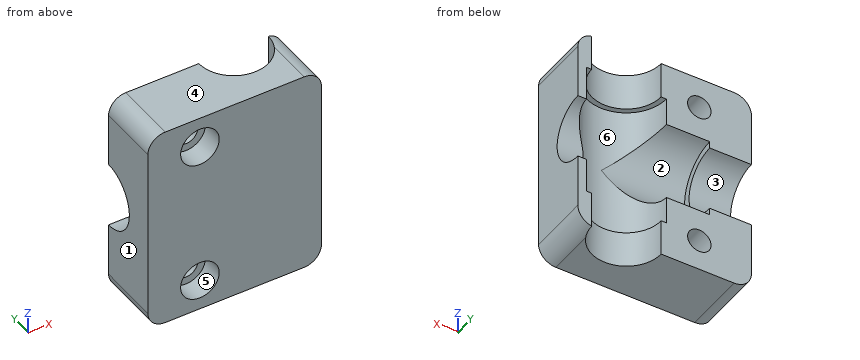
Autodesk Inventor part; units mm, degrees
ref_plane "Work Plane2" through (11, 18, -30) normal (1, 0, 0) x (0, 1, 0)
ref_plane "XZ Plane" through (0, 0, 0) normal (0, 1, 0) x (-1, 0, 0)
ref_plane "XY Plane" through (0, 0, 0) normal (0, 0, 1) x (1, 0, 0)
sketch "Sketch1" plane through (0, 0, 0) normal (0, 1, 0) x (-1, 0, 0)
  line L0 (-25, 30) -> (25, 30)
  line L1 (25, 30) -> (25, -30)
  line L2 (25, -30) -> (-25, -30)
  line L3 (-25, -30) -> (-25, 30)
  line L4 (-25, 30) -> (25, -30) construction
  line L5 (25, 30) -> (-25, -30) construction
  point P0 (0, 0)
  dimension "d0" = 50
  dimension "d1" = 60
extrude "Extrusion1" add sketch "Sketch1" along normal blind 18
sketch "Sketch2" plane through (25, 0, 30) normal (1, 0, 0) x (0, 0, -1)
  line L0 (60, 18) -> (0, 18)
  circle A0 centre (30, 18) radius 9.5
  point P0 (30, 0)
  point P1 (20.5, 18)
  point P2 (39.5, 18)
  dimension "d4" = 19
extrude "Extrusion2" cut sketch "Sketch2" against normal through all contours A0 L0 picked at (28.8771, 15.0391)
sketch "Sketch3" plane through (25, 0, -30) normal (0, 0, -1) x (-1, 0, 0)
  line L0 (0, 18) -> (50, 18)
  circle A0 centre (14, 18) radius 10
  point P0 (25, 0)
  point P1 (24, 18)
  point P2 (4, 18)
  dimension "d7" = 20
  dimension "d8" = 14
extrude "Extrusion3" cut sketch "Sketch3" against normal through all contours L0 A0 picked at (12.1065, 15.2567)
sketch "Sketch4" plane through (0, 0, 0) normal (0, 0, 1) x (1, 0, 0)
  arc A0 (1, 18) -> (21, 18) centre (11, 18) ccw
  circle A1 centre (11, 18) radius 11.5
  point P0 (0, 0)
  dimension "d11" = 23
extrude "Extrusion4" cut sketch "Sketch4" along normal mid plane 39
ref_plane "Work Plane2" through (11, 18, -30) normal (1, 0, 0) x (0, 1, 0)
sketch "Sketch5" plane through (11, 18, -30) normal (1, 0, 0) x (0, 1, 0)
  arc A0 (0, 39.5) -> (0, 20.5) centre (0, 30) ccw
  circle A1 centre (0, 30) radius 11.5
  point P0 (-18, 30)
  dimension "d14" = 23
extrude "Extrusion5" cut sketch "Sketch5" against normal blind 24
sketch "Sketch7" plane through (0, 0, 0) normal (0, -1, 0) x (1, 0, 0)
  line L0 (25, -30) -> (-25, -30)
  line L1 (-25, 30) -> (25, 30)
  line L2 (-25, -30) -> (-25, 30)
  point P0 (0, 0)
  point P1 (-10, -21)
  point P2 (-10, 21)
  dimension "d28" = 9
  dimension "d29" = 9
  dimension "d30" = 15
hole "Hole2" at (-10, 0, -21) at (-10, 0, 21) direction (0, 1, 0) diameter 6.756 end through all counterbore diameter 11.113 counterbore depth 6.35
fillet "Fillet1" radius 5 4 edges at (-25, 9, -30) (-25, 9, 30) (25, 9, 30) (25, 9, -30)
properties part number "Valve Block Bottom"
Source: CAD feature listing. Evaluate the final solid. Frame: model axes, mm. Face numbers are marked on the shaded views. A direction names the side the tool comes from. Give positions to 0.01 mm unless a question says otherwise; leave off trailing zeros. Order: outer loops, then holes, each group sorted by start corner. A loop starts at its lowest first (then second) coordinate and runs counter-clockwise, first axis right, second up.
(1) Section query D-D (y = 11.5). State how many separate pieces and enclosed holes the cut face has, plus the area to 3 significant figures.
(2) Material intervals for line 1 along Z through (x, y) = (-10, 3.5); line 2 along X through (y, z) = (4.5, -21); line 3 along Z through (x, y) = (-10, 9.75), sorted ascending.
(3) Pull-direction query (X, two-part tool) for the marked faces 1, 2 and 3; classes: +X half, -X half, draft (parallel to the pull), parting line (faces both ways), or undercut.
(4) Access query for the marked faces 4, 5 and 6. Directions: +Z, -Z, +X, -X, +Y, -Y. A direction counts if a zero-diameter tool reaches every point of the face in a straight line with its end or side. Return the directions, or none.
(5) Section query B-B (y = 2.5). Return the cut outline in (x, z).
(6) Section query A-A (z = -21). Return the cut outline in (x, y).
(7) Section query C-C (x = -10). Return the cut outline in (y, z), plus the area to 3 significant figures.
(8) Contact query for flat-ended pins moving along their axis: P1, Ø9, axis at y = 11.5, z = -5, coming from the +X side; P2, Ø9, axis at x = -10, z = 21, coming from the -Y side; P3, Ø1, axis at x = -12, z = -6.5, coming from the +Y side. Output: stop coordinate, or through.
Outcome:
1. separate pieces: 4
1. enclosed holes: 2
1. area: 1,340 mm2
2. line 1: z = -30 to -26.56, -15.44 to 15.44, 26.56 to 30
2. line 2: x = -25 to -15.56, -4.44 to 25
2. line 3: z = -30 to -24.38, -17.62 to -8.01, 8.01 to 17.62, 24.38 to 30
3. face 1: -X half
3. face 2: undercut
3. face 3: draft
4. face 4: +Z, +X, -X, +Y, -Y
4. face 5: -Y
4. face 6: +Y
5. outline: (-25, -25) arc R5 ccw to (-20, -30) - (20, -30) arc R5 ccw to (25, -25) - (25, 25) arc R5 ccw to (20, 30) - (-20, 30) arc R5 ccw to (-25, 25) - close; hole circle Ø11.11 at (-10, -21); hole circle Ø11.11 at (-10, 21)
6. outline: (-25, 0) - (-15.56, 0) - (-15.56, 6.35) - (-13.38, 6.35) - (-13.38, 18) - (-25, 18) - close; (-6.62, 6.35) - (-4.44, 6.35) - (-4.44, 0) - (25, 0) - (25, 18) - (21, 18) arc R10 cw to (1, 18) - (-6.62, 18) - close
7. outline: (0, -30) - (18, -30) - (18, -24.38) - (6.35, -24.38) - (6.35, -26.56) - (0, -26.56) - close; (0, -15.44) - (6.35, -15.44) - (6.35, -17.62) - (18, -17.62) - (18, -11.5) arc R11.5 cw to (18, 11.5) - (18, 17.62) - (6.35, 17.62) - (6.35, 15.44) - (0, 15.44) - close; (0, 26.56) - (6.35, 26.56) - (6.35, 24.38) - (18, 24.38) - (18, 30) - (0, 30) - close
7. area: 574 mm2
8. P1: stops at x = 25
8. P2: stops at y = 6.35
8. P3: stops at y = 8.88
